```python
from build123d import *

# Parameters (mm, degrees)
SKETCH1_R           = 2.05
SKETCH1_R_2         = 2.1
SKETCH1_R_3         = 1.9
SKETCH1_R_4         = 1.75
SKETCH1_R_5         = 1.95
SKETCH1_R_6         = 2
SKETCH1_R_7         = 1.8
SKETCH1_R_8         = 1.85
BOSS_EXTRUDE1_DEPTH = 4.2
BOSS_EXTRUDE2_DEPTH = 2
CHAMFER1_SIZE       = 0.5


with BuildPart() as part:
    # Sketch1 → Boss-Extrude1 (new body)
    with BuildSketch(Plane(origin=(0, 0, 0), x_dir=(1, 0, 0), z_dir=(0, 1, 0))):
        with BuildLine():
            Line((0, 5), (5, 0))
            Line((5, 0), (17.5, 0))
            ThreePointArc((17.5, 0), (19.267766953, 0.732233047), (20, 2.5))
            Line((20, 2.5), (20, 17.5))
            ThreePointArc((20, 17.5), (19.267766953, 19.267766953), (17.5, 20))
            Line((17.5, 20), (4, 20))
            ThreePointArc((4, 20), (1.171572875, 18.828427125), (0, 16))
            Line((0, 16), (0, 5))
        make_face()
        with Locations(Location((10, 4, 0), (0, 0, 270))):
            Circle(SKETCH1_R, mode=Mode.SUBTRACT)
        with Locations(Location((16, 4, 0), (0, 0, 270))):
            Circle(SKETCH1_R_2, mode=Mode.SUBTRACT)
        with Locations(Location((4, 10, 0), (0, 0, 270))):
            Circle(SKETCH1_R_3, mode=Mode.SUBTRACT)
        with Locations(Location((4, 16, 0), (0, 0, 270))):
            Circle(SKETCH1_R_4, mode=Mode.SUBTRACT)
        with Locations(Location((10, 10, 0), (0, 0, 270))):
            Circle(SKETCH1_R_5, mode=Mode.SUBTRACT)
        with Locations(Location((16, 10, 0), (0, 0, 270))):
            Circle(SKETCH1_R_6, mode=Mode.SUBTRACT)
        with Locations(Location((10, 16, 0), (0, 0, 270))):
            Circle(SKETCH1_R_7, mode=Mode.SUBTRACT)
        with Locations(Location((16, 16, 0), (0, 0, 270))):
            Circle(SKETCH1_R_8, mode=Mode.SUBTRACT)
    extrude(amount=BOSS_EXTRUDE1_DEPTH)

    # Sketch2 → Boss-Extrude2 (add)
    with BuildSketch(Plane(origin=(0, 4.2, 0), x_dir=(1, 0, 0), z_dir=(0, 1, 0))):
        with BuildLine():
            Line((20, 17.5), (20, 2.5))
            ThreePointArc((20, 2.5), (19.267766953, 0.732233047), (17.5, 0))
            Line((17.5, 0), (2.5, 0))
            ThreePointArc((2.5, 0), (0.732233047, 0.732233047), (0, 2.5))
            Line((0, 2.5), (0, 5))
            Line((0, 5), (0, 16))
            ThreePointArc((0, 16), (1.171572875, 18.828427125), (4, 20))
            Line((4, 20), (17.5, 20))
            ThreePointArc((17.5, 20), (19.267766953, 19.267766953), (20, 17.5))
        make_face()
    extrude(amount=BOSS_EXTRUDE2_DEPTH)

    # Chamfer1
    chamfer1_edges = [part.edges().sort_by_distance(p)[0] for p in [
        (19.267766953, 0, -19.267766953),
        (20, 0, -10),
        (19.267766953, 0, -0.732233047),
        (11.25, 0, 0),
        (2.5, 0, -2.5),
        (0, 0, -10.5),
        (1.171572875, 0, -18.828427125),
        (10.75, 0, -20),
        (4, 0, -17.75),
        (10, 0, -17.8),
        (16, 0, -17.85),
        (4, 0, -11.9),
        (10, 0, -11.95),
        (16, 0, -12),
        (10, 0, -6.05),
        (16, 0, -6.1),
    ]]
    chamfer(chamfer1_edges, length=CHAMFER1_SIZE)


solid = part.part
```
Geometry: final body of the model. Coordinates: model frame, mm. A direction names the side the tool comes from. Coordinates: 2 decimals unless noted, no trailing zeros. Order: outer loops, then holes, each group sorted by start corner. A loop starts at its lowest first (then second) coordinate and runs counter-clockwise, first axis right, second up. Notation, with made-up numbers: (81, 71.25) - (129, 71.25) arc R8 ccw to (129, 79.25) - close; hole circle Ø2 at (16, 9). An arc over 180 degrees is marked (long way). Return JSON: item names as keys, results as strings. Group by question number.
1. Cut plane A-A (x = 10). Output: boundary loops of the cut face in (y, z), plus the area to 3 significant figures.
2. Material intervals for line 1 along X through (y, z) = (2.35, -16); line 2 along X through (y, z) = (2.5, -4); line 3 along Z through (x, y) = (14.5, 1.75), sorted ascending. Write a range as [from, to].
3. Pull-direction query (X, two-part tool) for faces 3 (the face through (10, 4.2, -10)), 4 (the face through (2, 2, -3)), 5 (the face through (19.026, 0.135, -18.993)); classes: pulls with the +X half, pulls with the -X half, needs draft (parallel to the pull), parting line crosses it, or undercut.
4. Cut plane C-C (z = -4). Output: boundary loops of the cut face in (x, y).
5. Set-up query: faces 1 (the face through (19.248, 3.31, -19.287)), 2 (the face through (4, 4.2, -16)). Return all of +Z, -Z, +X, -X, +Y, -Y with unobstructed straight access to the full face (end or side cutting, diameter ignored); none if empty.
6. Cut plane D-D (x = 16). Output: boundary loops of the cut face in (y, z), plus the area to 3 significant figures.
7. Cut plane B-B (y = 1.25). Count the separate pieces of the cut face and the enclosed holes in it, plus the area to 3 significant figures.
8. Pin query (flat end, axial travel): pin 1 (1.8 mm diameter, centred on x = 9.5, z = -16, fed in from -Y); pin 2 (4 mm diameter, centred on x = 4, z = -10, fed in from -Y); pin 3 (2 mm diameter, centred on x = 3, z = -16, fed in from -Y). Return the tip coordinate at first contact, or that it passes through.
Resolved:
{
 "1": {"outline": "(0, -19.5) - (0.5, -20) - (6.2, -20) - (6.2, 0) - (0.5, 0) - (0, -0.5) - (0, -1.45) - (0.5, -1.95) - (4.2, -1.95) - (4.2, -6.05) - (0.5, -6.05) - (0, -6.55) - (0, -7.55) - (0.5, -8.05) - (4.2, -8.05) - (4.2, -11.95) - (0.5, -11.95) - (0, -12.45) - (0, -13.7) - (0.5, -14.2) - (4.2, -14.2) - (4.2, -17.8) - (0.5, -17.8) - (0, -18.3) - close", "area": "74.3 mm²"},
 "2": {"line 1": "x = [0, 2.25], [5.75, 8.2], [11.8, 14.15], [17.85, 20]", "line 2": "x = [1, 7.95], [12.05, 13.9], [18.1, 20]", "line 3": "z = [-20, -17.08], [-14.92, -11.32], [-8.68, -5.47], [-2.53, 0]"},
 "3": {"face 3": "undercut", "face 4": "pulls with the -X half", "face 5": "pulls with the +X half"},
 "4": {"outline": "(0, 4.2) - (1, 4.2) - (1, 0.5) - (1.71, 0) - (7.45, 0) - (7.95, 0.5) - (7.95, 4.2) - (12.05, 4.2) - (12.05, 0.5) - (12.55, 0) - (13.4, 0) - (13.9, 0.5) - (13.9, 4.2) - (18.1, 4.2) - (18.1, 0.5) - (18.6, 0) - (19.5, 0) - (20, 0.5) - (20, 6.2) - (0, 6.2) - close"},
 "5": {"face 1": "-Z, +X, +Y, -Y", "face 2": "-Y"},
 "6": {"outline": "(0, -19.5) - (0.5, -20) - (6.2, -20) - (6.2, 0) - (0.5, 0) - (0, -0.5) - (0, -1.4) - (0.5, -1.9) - (4.2, -1.9) - (4.2, -6.1) - (0.5, -6.1) - (0, -6.6) - (0, -7.5) - (0.5, -8) - (4.2, -8) - (4.2, -12) - (0.5, -12) - (0, -12.5) - (0, -13.65) - (0.5, -14.15) - (4.2, -14.15) - (4.2, -17.85) - (0.5, -17.85) - (0, -18.35) - close", "area": "73.0 mm²"},
 "7": {"separate pieces": "1", "enclosed holes": "8", "area": "288 mm²"},
 "8": {"pin 1": "stops at y = 4.2", "pin 2": "stops at y = 0.4", "pin 3": "stops at y = 0.25"}
}
